from build123d import *

# Parameters (mm, degrees)
F0_R          = 11.2999999997
F1_DEPTH      = 7.0000000005
F2_R          = 2.1333927031
F3_DEPTH      = 10.922
F3_DEPTH_BACK = 25.4
F4_R          = 2.1336
F5_DEPTH      = 10.922
F6_R          = 2.1336
F7_DEPTH      = 10.922
F8_R          = 2.1336
F9_DEPTH      = 10.922
F10_R         = 2.1336
F11_DEPTH     = 10.922
F12_R         = 2.1336
F13_DEPTH     = 10.922


with BuildPart() as f1:
    # F0 (on Top) → F1 (new body)
    with BuildSketch(Plane.XY):
        Polygon((14.6646968374, 33.8666666667), (0, 76.2), (-14.6646968374, 33.8666666667), (-43.9940905122, 0), (0, 8.4666666667), (43.9940905122, 0), align=None)
        with Locations((0, 25.4)):
            Circle(F0_R, mode=Mode.SUBTRACT)
    extrude(amount=F1_DEPTH)

    # F2 (on face) → F3 (cut, two sides)
    with BuildSketch(Plane(origin=(-1.5712175183, 8.1642857143, 0), x_dir=(0.9819805061, 0.1889822365, 0), z_dir=(0.1889822365, -0.9819805061, 0))) as f3_sk:
        with Locations((-26.335739265, 3.5000000002)):
            Circle(F2_R)
    extrude(amount=-F3_DEPTH, mode=Mode.SUBTRACT)
    extrude(f3_sk.sketch, amount=F3_DEPTH_BACK, mode=Mode.SUBTRACT)

    # F4 (on face) → F5 (cut)
    with BuildSketch(Plane(origin=(-25.1394802927, 21.7714285714, 0), x_dir=(-0.6546536707, -0.755928946, 0), z_dir=(-0.755928946, 0.6546536707, 0))):
        with Locations((11.9352928433, 3.5000000002)):
            Circle(F4_R)
    extrude(amount=-F5_DEPTH, mode=Mode.SUBTRACT)

    # F6 (on face) → F7 (cut)
    with BuildSketch(Plane(origin=(23.5682627744, 8.1642857143, 0), x_dir=(-0.3273268354, 0.9449111825, 0), z_dir=(0.9449111825, 0.3273268354, 0))):
        with Locations((55.1366321083, 3.5000000002)):
            Circle(F6_R)
    extrude(amount=-F7_DEPTH, mode=Mode.SUBTRACT)

    # F8 (on face) → F9 (cut)
    with BuildSketch(Plane(origin=(-23.5682627744, 8.1642857143, 0), x_dir=(-0.3273268354, -0.9449111825, 0), z_dir=(-0.9449111825, 0.3273268354, 0))):
        with Locations((-55.1397637729, 3.8250000005)):
            Circle(F8_R)
    extrude(amount=-F9_DEPTH, mode=Mode.SUBTRACT)

    # F10 (on face) → F11 (cut)
    with BuildSketch(Plane(origin=(25.1394802927, 21.7714285714, 0), x_dir=(-0.6546536707, 0.755928946, 0), z_dir=(0.755928946, 0.6546536707, 0))):
        with Locations((-11.938424508, 3.175)):
            Circle(F10_R)
    extrude(amount=-F11_DEPTH, mode=Mode.SUBTRACT)

    # F12 (on face) → F13 (cut)
    with BuildSketch(Plane(origin=(1.5712175183, 8.1642857143, 0), x_dir=(0.9819805061, -0.1889822365, 0), z_dir=(-0.1889822365, -0.9819805061, 0))):
        with Locations((26.3388709296, 3.8250000005)):
            Circle(F12_R)
    extrude(amount=-F13_DEPTH, mode=Mode.SUBTRACT)


solid = f1.part
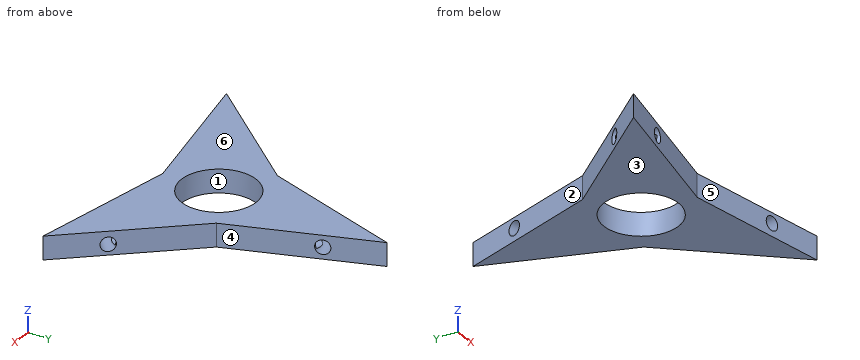
Design review of the part built by this model. Coordinates are the model's own, in mm. Face numbers are marked on the shaded views. A direction names the side the tool comes from. Round coordinates to 2 decimals unless told otherwise and drop trailing zeros. Order: outer loops, then holes, each group sorted by start corner. A loop starts at its lowest first (then second) coordinate and runs counter-clockwise, first axis right, second up.
1) Consider section A-A (x = -8.5). State the section outline as (y, z) points, plus the area to 3 significant figures.
The answers:
outline: (6.83, 0) - (17.95, 0) - (17.95, 7) - (6.83, 7) - close; (32.85, 0) - (51.66, 0) - (51.66, 7) - (32.85, 7) - close
area: 210 mm2
2) Consider section B-B (y = 25.4). State the section outline as (x, z) points, plus the area to 3 significant figures.
The answers:
outline: (-22, 0) - (-11.3, 0) - (-11.3, 7) - (-22, 7) - close; (11.3, 0) - (22, 0) - (22, 7) - (11.3, 7) - close
area: 150 mm2
3) Machinability: for the marked faces 5 and 6, which of the approach directions +Z, -Z, +X, -X, +Y, -Y give a long, thin tool a straight path to every point of the face, cutting with its end or side? Answer none if there is none.
The answers:
face 5: +Z, -Z, -Y
face 6: +Z, +X, -X, +Y, -Y
4) Clearance check with flat-ended pins moving along their axes: pin 1 Ø8 at (x, y) = (-18, 48) entering from +Z; pin 2 Ø2 at (y, z) = (44.5, 3.5) entering from +X; pin 3 Ø1 at (y, z) = (40, 1) entering from -X; pin 4 Ø6 at (x, y) = (11.5, 30.5) entering from -Z. State where each tip first meets the part, or that it passes through.
The answers:
pin 1: passes through
pin 2: stops at x = 11.33
pin 3: stops at x = -12.71
pin 4: stops at z = 0
5) Consider section D-D (x = 38). State the section outline as (y, z) points, plus the area to 3 significant figures.
The answers:
outline: (1.15, 0) - (6.92, 0) - (6.92, 7) - (1.15, 7) - close
area: 40.4 mm2
6) Consider section C-C (y = 46). State the section outline as (x, z) points.
The answers:
outline: (-10.46, 0) - (10.46, 0) - (10.46, 7) - (-10.46, 7) - close
7) Draft analysis for pull direction X (two halves, no side actions). For the marked faces 1, 2, 3 and 4, state which applies: released by +X, released by -X, zero draft, split by the parting line, or undercut.
The answers:
face 1: undercut
face 2: released by -X
face 3: zero draft
face 4: released by +X
8) For L1, parallel to Y at x = -31, z = 3.25; L2, parallel to X at y = 17, z = 6; L3, parallel to Y at x = 31.5, z = 2.75, list the stretches that pass through material, from the lowest coordinate up.
The answers:
L1: y = 2.5 to 8.25, 13.86 to 15
L2: x = -29.27 to -7.56, 7.56 to 29.27
L3: y = 2.4 to 8.72, 14.25 to 14.43
